Autodesk Inventor part; units mm, degrees
ref_plane "Work Plane1" through (-11, -5, -8) normal (0, 0, -1) x (0, 1, 0)
ref_plane "YZ Plane" through (0, 0, 0) normal (1, 0, 0) x (0, 1, 0)
ref_plane "XZ Plane" through (0, 0, 0) normal (0, 1, 0) x (-1, 0, 0)
sketch "Sketch1" plane through (0, 0, 0) normal (0, 0, 1) x (1, 0, 0)
  arc A0 (5, -5) -> (-5, -5) centre (0, -5) ccw
  circle A1 centre (0, -5) radius 5
  arc A2 (4.3589, 4) -> (-4.3589, 4) centre (0, -5) ccw
  line L0 (12, -5) -> (12, 4)
  line L1 (11, 4) -> (4.3589, 4)
  line L2 (12, 4) -> (0, 4)
  line L3 (0, 4) -> (0, -5)
  line L4 (0, -5) -> (12, -5)
  line L5 (12, -5) -> (12, 4)
  arc A3 (-4.3589, -14) -> (4.3589, -14) centre (0, -5) ccw
  line L6 (12, -5) -> (12, -14)
  line L7 (12, -14) -> (0, -14)
  line L8 (-12, -5) -> (-12, 4)
  line L9 (-12, 4) -> (0, 4)
  line L10 (0, -5) -> (-12, -5)
  line L11 (-12, -14) -> (0, -14)
  line L12 (-12, -5) -> (-12, -14)
  circle A4 centre (0, -5) radius 10
  point P0 (0, 0)
ref_plane "Work Plane1" through (-11, -5, -8) normal (0, 0, -1) x (0, 1, 0)
extrude "Extrusion1" add sketch "Sketch1" against normal up to surface (8 mm away) contours L4 A4 L7 L11 L10 A1 | L4 L6 L7 A4 | A4 L11 L12 L10 | A3 L11 L7
sketch "Sketch2" plane through (4.3589, -14, 0) normal (0, -1, 0) x (1, 0, 0)
  circle A0 centre (3.8206, -4) radius 1.7
  circle A1 centre (-12.5383, -4) radius 1.7
  point P0 (-4.3589, 0)
hole "Hole1" at (-8.1794, -14, -4) at (8.1794, -14, -4) direction (0, 1, 0) diameter 3.4 end through all counterbore diameter 6.5 counterbore depth 3
fillet "Fillet1" radius 1 2 edges at (12, -9.5, 0) (-12, -9.5, 0)
sketch "Sketch3" plane through (0, 0, 0) normal (0, 0, 1) x (1, 0, 0)
  line L0 (-8, 4.75) -> (11, 4.75)
  line L1 (-8, 4.75) -> (-8, -5)
  line L2 (-8, -5) -> (-5, -5)
  arc A0 (-4.7896, -3.5647) -> (-5, -5) centre (0, -5) ccw
  line L3 (-4.7896, -3.5647) -> (-4.0711, -3.78)
  line L4 (-4.0711, -3.78) -> (-3.7492, -2.9985)
  line L5 (-3.7492, -2.9985) -> (-4.4108, -2.6453)
  arc A1 (-3.185, -1.1457) -> (-4.4108, -2.6453) centre (0, -5) ccw
  line L6 (-3.185, -1.1457) -> (-2.7072, -1.7238)
  line L7 (-2.7072, -1.7238) -> (-2.0054, -1.2529)
  line L8 (-2.0054, -1.2529) -> (-2.3593, -0.5916)
  arc A2 (-0.5069, -0.0258) -> (-2.3593, -0.5916) centre (0, -5) ccw
  line L9 (-0.5069, -0.0258) -> (-0.4308, -0.7719)
  line L10 (-0.4308, -0.7719) -> (0.4144, -0.7702)
  line L11 (0.4144, -0.7702) -> (0.4875, -0.0238)
  arc A3 (2.3421, -0.5825) -> (0.4875, -0.0238) centre (0, -5) ccw
  line L12 (2.3421, -0.5825) -> (1.9908, -1.2451)
  line L13 (1.9908, -1.2451) -> (2.6945, -1.7133)
  line L14 (2.6945, -1.7133) -> (3.17, -1.1333)
  arc A4 (4.4016, -2.6282) -> (3.17, -1.1333) centre (0, -5) ccw
  line L15 (4.4016, -2.6282) -> (3.7414, -2.9839)
  line L16 (3.7414, -2.9839) -> (4.0664, -3.7642)
  line L17 (4.0664, -3.7642) -> (4.7839, -3.5461)
  arc A5 (5, -5) -> (4.7839, -3.5461) centre (0, -5) ccw
  line L18 (5, -5) -> (11, -5)
  line L19 (11, 4.75) -> (11, -5)
  circle A6 centre (0, -5) radius 5
  line L20 (-4.7896, -6.4353) -> (-4.0711, -6.22)
  line L21 (-4.0711, -6.22) -> (-3.7492, -7.0015)
  line L22 (-3.7492, -7.0015) -> (-4.4108, -7.3547)
  arc A7 (-4.4108, -7.3547) -> (-3.185, -8.8543) centre (0, -5) ccw
  line L23 (-3.185, -8.8543) -> (-2.7072, -8.2762)
  line L24 (-2.7072, -8.2762) -> (-2.0054, -8.7471)
  line L25 (-2.0054, -8.7471) -> (-2.3593, -9.4084)
  arc A8 (-2.3593, -9.4084) -> (-0.5069, -9.9742) centre (0, -5) ccw
  line L26 (-0.5069, -9.9742) -> (-0.4308, -9.2281)
  line L27 (-0.4308, -9.2281) -> (0.4144, -9.2298)
  line L28 (0.4144, -9.2298) -> (0.4875, -9.9762)
  arc A9 (0.4875, -9.9762) -> (2.3421, -9.4175) centre (0, -5) ccw
  line L29 (2.3421, -9.4175) -> (1.9908, -8.7549)
  line L30 (1.9908, -8.7549) -> (2.6945, -8.2867)
  line L31 (2.6945, -8.2867) -> (3.17, -8.8667)
  arc A10 (3.17, -8.8667) -> (4.4016, -7.3718) centre (0, -5) ccw
  line L32 (4.4016, -7.3718) -> (3.7414, -7.0161)
  line L33 (3.7414, -7.0161) -> (4.0664, -6.2358)
  line L34 (4.0664, -6.2358) -> (4.7839, -6.4539)
  point P0 (0, 0)
  point P1 (0, -10)
  point P2 (-4.4108, -7.3547)
  point P3 (-0.5069, -9.9742)
  point P4 (2.3421, -9.4175)
  point P5 (4.4016, -7.3718)
extrude "Extrusion2" add sketch "Sketch3" against normal blind 1 contours L20 L21 L22 A6 | A6 L32 L33 L34 | L23 L24 L25 A6 | A6 L29 L30 L31 | L26 L27 L28 A6
pattern_linear "Rectangular Pattern1" count 3 spacing 3.5 along (0, 0, -1) of "Extrusion2"
properties part number "Bed Cable Harness Cable Clamp"
Geometry: final body of the model. Coordinates: model frame, mm. A direction names the side the tool comes from. Coordinates: 2 decimals unless noted, no trailing zeros. Order: outer loops, then holes, each group sorted by start corner. A loop starts at its lowest first (then second) coordinate and runs counter-clockwise, first axis right, second up. Notation, with made-up numbers: (29.5, 17) - (68.5, 17) arc R27 ccw to (68.5, 34) - close; hole circle Ø10 at (87.25, 71). An arc over 180 degrees is marked (long way). Return JSON: item names as keys, results as strings. Group by question number.
1. Cut plane C-C (z = -4.75). Output: boundary loops of the cut face in (x, y).
2. Set-up query: faces 4 (the face through (11.063, -12.479, -5.5)), 5 (the face through (12, -9, -4)), 6 (the face through (-4.3, -6.8, -7)). Return all of +Z, -Z, +X, -X, +Y, -Y with unobstructed straight access to the full face (end or side cutting, diameter ignored); none if empty.
3. Cut plane D-D (x = 0). Output: boundary loops of the cut face in (y, z), plus the area to 3 significant figures.
4. Pin query (flat end, axial travel): pin 1 (2.5 mm diameter, centred on x = 8.5, z = -3, fed in from -Y); pin 2 (2 mm diameter, centred on x = 3.5, z = -5, fed in from -Y). Return the tip coordinate at first contact, or that it passes through.
5. Material intervals for line 1 along X through (y, z) = (-7.9, -4); line 2 along X through (y, z) = (-8.1, -4); line 3 along X through (y, z) = (-13.75, -5), sorted ascending. Write a range as [from, to].
6. Cut plane A-A (x = -6.75). Output: boundary loops of the cut face in (y, z).
7. Cut plane B-B (y = -13.25). Output: boundary loops of the cut face in (x, z).
8. Pull-direction query (Z, two-part tool) for faces 1 (the face through (-11.699, -9.563, -0.285)), 2 (the face through (-11.6, -14, -3.9)), 3 (the face through (10, -11, -5)); classes: pulls with the +Z half, pulls with the -Z half, needs draft (parallel to the pull), parting line crosses it, or undercut.
Resolved:
{
 "1": {"outline": "(-12, -14) - (-11.34, -14) - (-11.34, -11) - (-9.71, -11) - (-9.71, -5) - (-12, -5) - close; (-6.65, -11) - (-5.02, -11) - (-5.02, -14) - (-4.36, -14) arc R10 ccw to (4.36, -14) - (5.02, -14) - (5.02, -11) - (6.65, -11) - (6.65, -5) - (5, -5) arc R5 cw to (-5, -5) - (-6.65, -5) - close; (9.71, -11) - (11.34, -11) - (11.34, -14) - (12, -14) - (12, -5) - (9.71, -5) - close"},
 "2": {"face 4": "-Y", "face 5": "+Z, -Z, +X, +Y, -Y", "face 6": "+Y"},
 "3": {"outline": "(-15, -8) - (-9.23, -8) - (-9.23, -7) - (-10, -7) - (-10, -4.5) - (-9.23, -4.5) - (-9.23, -3.5) - (-10, -3.5) - (-10, -1) - (-9.23, -1) - (-9.23, 0) - (-15, 0) - close", "area": "42.3 mm²"},
 "4": {"pin 1": "stops at y = -11", "pin 2": "stops at y = -14.68"},
 "5": {"line 1": "x = [-12, -9.88], [-6.48, -4.07], [4.07, 6.48], [9.88, 12]", "line 2": "x = [-12, -9.88], [-6.48, -3.92], [3.92, 6.48], [9.88, 12]", "line 3": "x = [-12, -11.27], [-5.09, 5.09], [11.27, 12]"},
 "6": {"outline": "(-14, -8) - (-5, -8) - (-5, -4.92) - (-11, -4.92) - (-11, -6.92) - (-14, -6.92) - close; (-14, -1.08) - (-11, -1.08) - (-11, -3.08) - (-5, -3.08) - (-5, 0) - (-14, 0) - close"},
 "7": {"outline": "(-12, -8) - (12, -8) - (12, -1) arc R1 ccw to (11, 0) - (-11, 0) arc R1 ccw to (-12, -1) - close; hole circle Ø6.5 at (-8.18, -4); hole circle Ø6.5 at (8.18, -4)"},
 "8": {"face 1": "pulls with the +Z half", "face 2": "needs draft", "face 3": "undercut"}
}
